Can you work these out from the model? Positions are in its coordinate system, mm. Face numbers are marked on the shaded views. A direction names the side the tool comes from. Give positions to 0.01 mm unless a question says otherwise; leave off trailing zeros. Write each loop counter-clockwise with the first axis right and the second up, starting at its lowest first coordinate (ties: lowest second). Pieces come first, ordered by that corner, then holes. Notation, with made-up numbers: (60.25, -34.75) - (97.25, -34.75) arc R20 cw to (97.25, -28.75) - close; hole circle Ø10 at (49, -11). An arc over 180 degrees is marked (long way). Return JSON: item names as keys, results as strings. Group by question number.
from build123d import *

# Parameters (mm, degrees)
EXTRUDE_1_DEPTH     = 15
SKETCH_4_W          = 1.562441002
SKETCH_4_H          = 15
SKETCH_4_W_2        = 6.177038061
EXTRUDE_3_DEPTH     = 5
SKETCH_2_R          = 6.01
CUT_EXTRUDE_2_DEPTH = 200
SKETCH_7_W          = 3.025917145
SKETCH_7_H          = 15
EXTRUDE_4_DEPTH     = 46.224
FILLET_1_R          = 2
FILLET_2_R          = 5
SKETCH_8_W          = 7.260520937
SKETCH_8_H          = 15
SKETCH_8_R          = 2
SKETCH_8_W_2        = 19.713561918
SKETCH_8_W_3        = 3.025917145
EXTRUDE_5_DEPTH     = 2


with BuildPart() as part:
    # 草图1 → 凸台-拉伸1 (new body)
    with BuildSketch(Plane(origin=(0, 0, 0), x_dir=(1, 0, 0), z_dir=(0, 1, 0))):
        with BuildLine():
            Line((-10.28806108, -6.177038061), (-10.28806108, 6.177038061))
            ThreePointArc((-10.28806108, 6.177038061), (12, 0), (-10.28806108, -6.177038061))
        make_face()
    extrude(amount=EXTRUDE_1_DEPTH)

    # 草图4 → 凸台-拉伸3 (add)
    with BuildSketch(Plane.ZY.offset(10.28806108)):
        with Locations((6.958258562, 7.5)):
            Rectangle(SKETCH_4_W, SKETCH_4_H)
        with Locations((-6.958258562, 7.5)):
            Rectangle(SKETCH_4_W, SKETCH_4_H)
        with Locations((-3.088519031, 7.5)):
            Rectangle(SKETCH_4_W_2, SKETCH_4_H)
        with Locations((3.088519031, 7.5)):
            Rectangle(SKETCH_4_W_2, SKETCH_4_H)
    extrude(amount=-EXTRUDE_3_DEPTH)

    # 草图2 → 切除-拉伸2 (cut)
    with BuildSketch(Plane(origin=(0, 15, 0), x_dir=(1, 0, 0), z_dir=(0, 1, 0))):
        with Locations(Location((0, 0, 0), (0, 0, 270))):
            Circle(SKETCH_2_R)
    extrude(amount=-CUT_EXTRUDE_2_DEPTH, mode=Mode.SUBTRACT)

    # 草图7 → 凸台-拉伸4 (add)
    with BuildSketch(Plane.ZY.offset(10.28806108)):
        with Locations((6.226520491, 7.5)):
            Rectangle(SKETCH_7_W, SKETCH_7_H)
        with Locations((-6.226520491, 7.5)):
            Rectangle(SKETCH_7_W, SKETCH_7_H)
    extrude(amount=EXTRUDE_4_DEPTH)

    # 圆角1
    fillet_1_edges = [part.edges().sort_by_distance(p)[0] for p in [
        (-10.28806108, 7.5, 4.713561918),
        (-10.28806108, 7.5, -4.713561918),
    ]]
    fillet(fillet_1_edges, radius=FILLET_1_R)

    # 圆角2
    fillet_2_edges = [part.edges().sort_by_distance(p)[0] for p in [
        (-9.170630504, 7.5, -7.739479063),
        (-9.170630504, 7.5, 7.739479063),
    ]]
    fillet(fillet_2_edges, radius=FILLET_2_R)

    # 草图8 → 凸台-拉伸5 (add)
    # profile 1 of 3: a face of its own
    with BuildSketch(Plane.ZY.offset(56.51206108)):
        with Locations((11.369739532, 7.5)):
            Rectangle(SKETCH_8_W, SKETCH_8_H)
        with Locations((12, 7.5)):
            Circle(SKETCH_8_R, mode=Mode.SUBTRACT)
    # profile 2 of 3: a face of its own
    with BuildSketch(Plane.ZY.offset(56.51206108)):
        with Locations((-5.143219041, 7.5)):
            Rectangle(SKETCH_8_W_2, SKETCH_8_H)
        with Locations((-12, 7.5)):
            Circle(SKETCH_8_R, mode=Mode.SUBTRACT)
    # profile 3 of 3: a face of its own
    with BuildSketch(Plane.ZY.offset(56.51206108)):
        with Locations((6.226520491, 7.5)):
            Rectangle(SKETCH_8_W_3, SKETCH_8_H)
    extrude(amount=EXTRUDE_5_DEPTH)


solid = part.part
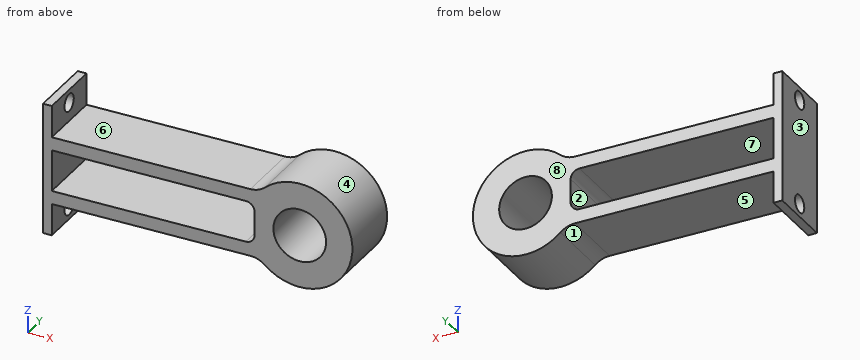
1) I need wall thicknesses on line 1 along Z through (x, y) = (-28, 7.25); line 2 along Y through (x, z) = (-57.2, -12); line 3 along X through (y, z) = (8.5, 0). Which ranges of each line are inside material? Lowest first, please.
2) Imagine slicing it at D-D, the plane y = 12.5. Write out the boundary of the cut face in (x, z).
3) Imagine slicing it at B-B, the plane x = -15.5. Write out the boundary of the cut face in (y, z), and give its area (3 significant figures).
4) Will these pins go through, and if not, where does the flat tip stop? pin 1 Ø4.5 at (x, y) = (-24, 11) entering from +Z; pin 2 Ø8 at (y, z) = (7.5, -5.5) entering from +X; pin 3 Ø6 at (y, z) = (5, 9.5) entering from +X.
5) On a 3-axis mill with a long thin cutter (end or side, diameter ignored), from which of +Z, -Z, +X, -X, +Y, -Y can I reach the whole of each face in a straight line? I mean the marked faces 5, 6, 7 and 8. Say none if no direction works.
6) We'd pull the mould along Z, two halves only. Please class the marked faces 1, 2, 3 and 4: pulls with the +Z half, pulls with the -Z half, needs draft (parallel to the pull), parting line crosses it, or undercut.
7) Imagine slicing it at C-C, the plane z = -4. Write out the boundary of the cut face in (x, y), and give its area (3 significant figures).
8) Imagine slicing it at A-A, the plane y = 7.5. Write out the boundary of the cut face in (x, z), and give its area (3 significant figures).
Resolved:
{
 "1": {"line 1": "-7.74 to -4.71, 4.71 to 7.74", "line 2": "0 to 5.5, 9.5 to 15", "line 3": "-58.51 to -56.51, -10.29 to -6.01, 6.01 to 12"},
 "2": {"outline": "(-58.51, -15) - (-56.51, -15) - (-56.51, -7.74) - (-11.26, -7.74) arc R5 cw to (-7.95, -8.99) arc R12 ccw (long way) to (-7.95, 8.99) arc R5 cw to (-11.26, 7.74) - (-56.51, 7.74) - (-56.51, 15) - (-58.51, 15) - close; hole (-56.51, -4.71) - (-12.29, -4.71) arc R2 ccw to (-10.29, -2.71) - (-10.29, 2.71) arc R2 ccw to (-12.29, 4.71) - (-56.51, 4.71) - close; hole circle Ø12.02 at (0, 0)"},
 "3": {"outline": "(0, -7.74) - (15, -7.74) - (15, -4.71) - (0, -4.71) - close; (0, 4.71) - (15, 4.71) - (15, 7.74) - (0, 7.74) - close", "area": "90.8 mm^2"},
 "4": {"pin 1": "z = 7.74", "pin 2": "x = 11.91", "pin 3": "x = 10.09"},
 "5": {"face 5": "-Z, +Y, -Y", "face 6": "+Z, +Y, -Y", "face 7": "+Y, -Y", "face 8": "+Z, -Z, +X, -X, +Y"},
 "6": {"face 1": "pulls with the -Z half", "face 2": "undercut", "face 3": "needs draft", "face 4": "parting line crosses it"},
 "7": {"outline": "(-58.51, 0) - (-56.51, 0) - (-56.51, 15) - (-58.51, 15) - close; (-10.76, 0) - (-4.49, 0) - (-4.49, 15) - (-10.76, 15) - close; (4.49, 0) - (11.31, 0) - (11.31, 15) - (4.49, 15) - close", "area": "226 mm^2"},
 "8": {"outline": "(-58.51, -15) - (-56.51, -15) - (-56.51, -14) - (-58.51, -14) - close; (-58.51, -10) - (-56.51, -10) - (-56.51, -7.74) - (-11.26, -7.74) arc R5 cw to (-7.95, -8.99) arc R12 ccw (long way) to (-7.95, 8.99) arc R5 cw to (-11.26, 7.74) - (-56.51, 7.74) - (-56.51, 10) - (-58.51, 10) - close; (-58.51, 14) - (-56.51, 14) - (-56.51, 15) - (-58.51, 15) - close; hole (-56.51, -4.71) - (-12.29, -4.71) arc R2 ccw to (-10.29, -2.71) - (-10.29, 2.71) arc R2 ccw to (-12.29, 4.71) - (-56.51, 4.71) - close; hole circle Ø12.02 at (0, 0)", "area": "653 mm^2"}
}
